Study the drawing (mm; zero at the part's minimum x, y, z) and answer. A direction names the side the tool comes from. Round coordinates to 2 decimals unless told otherwise and drop trailing zeros. Write each loop counter-clockwise with the first axis right and the second up, starting at its lowest first coordinate (ties: lowest second). Pieces come first, ordered by that corner, then holes. Notation, with made-up numbers: (28, -27) - (47, -27) arc R16 cw to (47, 1) - close; hole circle Ø9 at (38.5, 53). An arc over 180 degrees is marked (long way). Use one line per item in the form item = value. Start each with the question number.
1) For a pull along X with two mould halves and no side action, classify the marked faces 3, 4, 5 and 6 as released by +X, released by -X, zero draft, split by the parting line, or undercut.
2) Each of these flat-tipped pins is pushed along its axis until it touches: pin 1 (1.5 mm diameter, centred on x = 4, z = 21, fed in from +Y); pin 2 (1.5 mm diameter, centred on y = 21, z = 10.5, fed in from -X) (1 decimal); pin 3 (12 mm diameter, centred on x = 24, z = 9.5, fed in from +Y). Where does it stop, or does it pass through?
3) The part is cut by section D-D, the plane y = 24.5. Give the vertices of the cut face in (x, z).
4) For the marked faces 1 and 2, determine the directions among +Z, -Z, +X, -X, +Y, -Y from which every point of the face is accessible in a straight line to the end or side of a thin tool.
5) Consider line 1 along Y through (x, z) = (22, 10) (1 decimal); line 2 along X through (y, z) = (12, 11.5); line 3 along Y through (x, z) = (17, 16.5). Determine where each line is inside the solid, lowest interval first. Write a range as from..to.
6) The part is cut by section B-B, the plane y = 15. Give the vertices of the cut face in (x, z), plus the area to 3 significant figures.
7) The part is cut by section C-C, the plane x = 7. Give the vertices of the cut face in (y, z).
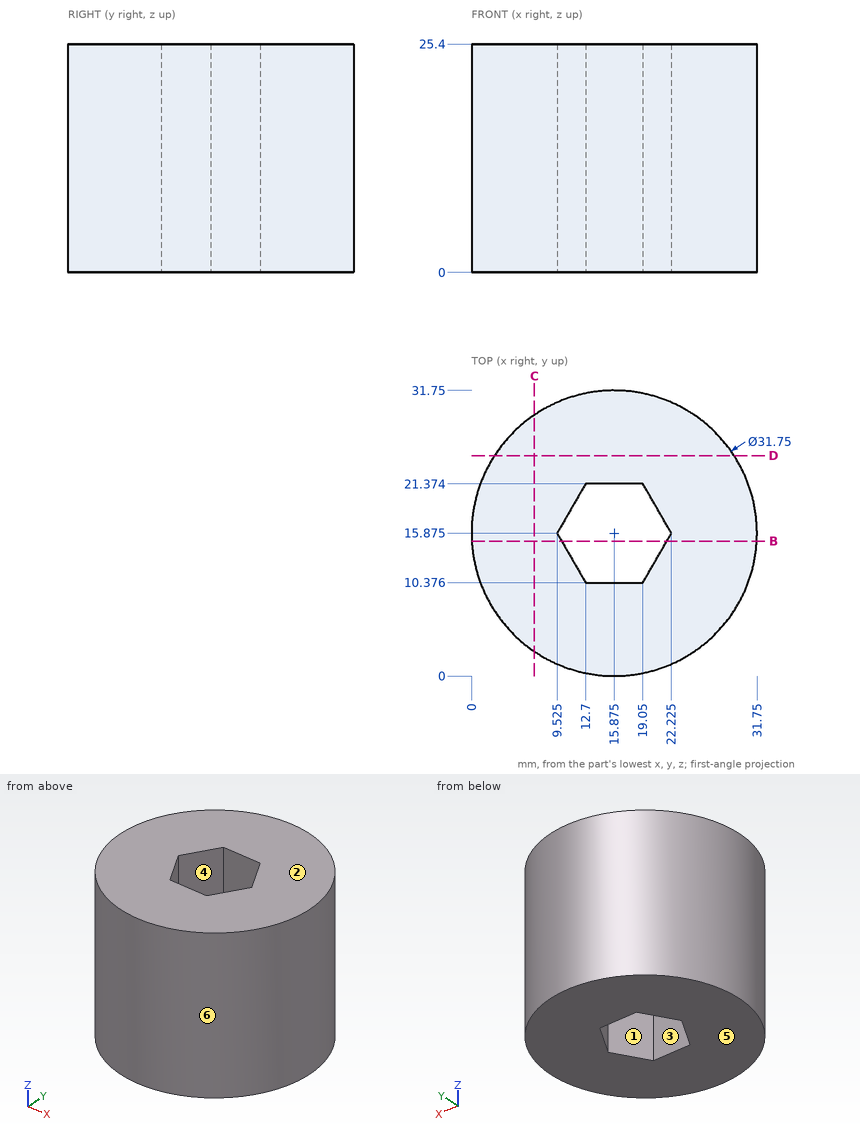
Geometry results:
q1.face_3 = undercut
q1.face_4 = undercut
q1.face_5 = zero draft
q1.face_6 = split by the parting line
q2.pin_1 = 27.2
q2.pin_2 = 0.6
q2.pin_3 = 31.61
q3.outline = (2.55, 0) - (29.2, 0) - (29.2, 25.4) - (2.55, 25.4) - close
q4.face_1 = +Z, -Z
q4.face_2 = +Z, +X, -X, +Y, -Y
q5.line_1 = 1.2..15.5, 16.3..30.5
q5.line_2 = 0.48..11.76, 19.99..31.27
q5.line_3 = 0.04..10.38, 21.37..31.71
q6.outline = (0.02, 0) - (10.03, 0) - (10.03, 25.4) - (0.02, 25.4) - close; (21.72, 0) - (31.73, 0) - (31.73, 25.4) - (21.72, 25.4) - close
q6.area = 508 mm2
q7.outline = (2.71, 0) - (29.04, 0) - (29.04, 25.4) - (2.71, 25.4) - close
